Read the model definition and answer for the solid it produces. Units are mm, in the model's axes. Face numbers are marked on the shaded views. A direction names the side the tool comes from. Give positions to 0.01 mm unless a question says otherwise; leave off trailing zeros. Order: outer loops, then holes, each group sorted by start corner. A loop starts at its lowest first (then second) coordinate and runs counter-clockwise, first axis right, second up.
```python
from build123d import *

# Parameters (mm, degrees)
F0_R     = 2.25
F0_R_2   = 33.35
F1_DEPTH = 20
F2_R     = 33.35
F3_DEPTH = 25
F5_DEPTH = 5
F6_R     = 1.49999
F7_SIZE  = 5
F8_R     = 1.99999


# Not quite as in the source:
# - a fillet or chamfer is up to 0.001 mm smaller than in the source, because OpenCascade refuses the exact size


with BuildPart() as f1:
    # F0 (on Top) → F1 (new body)
    with BuildSketch(Plane.XY):
        with BuildLine():
            ThreePointArc((-35.3461431703, -28.7786841774), (-30.3488782685, -27.4389385893), (-25.3508812473, -28.775950375))
            ThreePointArc((-25.3508812473, -28.775950375), (0, -38.35), (25.3508812473, -28.775950375))
            ThreePointArc((25.3508812473, -28.775950375), (30.3488782685, -27.4389385893), (35.3461431703, -28.7786841774))
            ThreePointArc((35.3461431703, -28.7786841774), (45.2498273477, -26.125), (42.5961431703, -16.2213158226))
            ThreePointArc((42.5961431703, -16.2213158226), (38.9372570055, -12.5634302623), (37.5961446665, -7.566531981))
            ThreePointArc((37.5961446665, -7.566531981), (33.2120742351, 19.175), (12.2452634191, 36.342482356))
            ThreePointArc((12.2452634191, 36.342482356), (8.588378737, 40.0023688516), (7.25, 45))
            ThreePointArc((7.25, 45), (5.790617411, 49.3624820917), (2, 51.9686799324))
            Line((2, 51.9686799324), (2, 54.1277186767))
            Line((2, 54.1277186767), (2, 57))
            Line((2, 57), (0, 57))
            Line((0, 57), (-2, 57))
            Line((-2, 57), (-2, 54.1277186767))
            Line((-2, 54.1277186767), (-2, 51.9686799324))
            ThreePointArc((-2, 51.9686799324), (-5.790617411, 49.3624820917), (-7.25, 45))
            ThreePointArc((-7.25, 45), (-8.588378737, 40.0023688516), (-12.2452634191, 36.342482356))
            ThreePointArc((-12.2452634191, 36.342482356), (-33.2120742351, 19.175), (-37.5961446665, -7.566531981))
            ThreePointArc((-37.5961446665, -7.566531981), (-38.9372570055, -12.5634302623), (-42.5961431703, -16.2213158226))
            ThreePointArc((-42.5961431703, -16.2213158226), (-45.2498273477, -26.125), (-35.3461431703, -28.7786841774))
        make_face()
        with Locations((-38.9711431703, -22.5)):
            Circle(F0_R, mode=Mode.SUBTRACT)
        with Locations((38.9711431703, -22.5)):
            Circle(F0_R, mode=Mode.SUBTRACT)
        Circle(F0_R_2, mode=Mode.SUBTRACT)
        with Locations((0, 45)):
            Circle(F0_R, mode=Mode.SUBTRACT)
    extrude(amount=F1_DEPTH)

    # F2 (on Top) → F3 (join)
    with BuildSketch(Plane.XY):
        Polygon((37.0225860118, -21.375), (37.0225860118, 21.375), (0, 42.75), (-37.0225860118, 21.375), (-37.0225860118, -21.375), (0, -42.75), align=None)
        Circle(F2_R, mode=Mode.SUBTRACT)
    extrude(amount=F3_DEPTH)

    # F4 (on face) → F5 (cut)
    with BuildSketch(Plane.XY.offset(25)):
        Polygon((37.0225860118, -21.375), (37.0225860118, 21.375), (0, 42.75), (-37.0225860118, 21.375), (-37.0225860118, -21.375), (0, -42.75), align=None)
        with BuildLine():
            ThreePointArc((-31.7698222916, -16.6102646446), (-31.0470107257, 17.925), (-1.5, 35.8186055005))
            Line((-1.5, 35.8186055005), (-1.5, 38.8186055005))
            Line((-1.5, 38.8186055005), (0, 38.8186055005))
            Line((0, 38.8186055005), (1.5, 38.8186055005))
            Line((1.5, 38.8186055005), (1.5, 35.8186055005))
            ThreePointArc((1.5, 35.8186055005), (31.0470107257, 17.925), (31.7698222916, -16.6102646446))
            Line((31.7698222916, -16.6102646446), (34.3678985029, -18.1102646446))
            Line((34.3678985029, -18.1102646446), (33.6178985029, -19.4093027502))
            Line((33.6178985029, -19.4093027502), (32.8678985029, -20.7083408559))
            Line((32.8678985029, -20.7083408559), (30.2698222916, -19.2083408559))
            ThreePointArc((30.2698222916, -19.2083408559), (0, -35.85), (-30.2698222916, -19.2083408559))
            Line((-30.2698222916, -19.2083408559), (-32.8678985029, -20.7083408559))
            Line((-32.8678985029, -20.7083408559), (-33.6178985029, -19.4093027502))
            Line((-33.6178985029, -19.4093027502), (-34.3678985029, -18.1102646446))
            Line((-34.3678985029, -18.1102646446), (-31.7698222916, -16.6102646446))
        make_face(mode=Mode.SUBTRACT)
    extrude(amount=-F5_DEPTH, mode=Mode.SUBTRACT)

    # F6 (radius 1.5 in the source; OpenCascade refuses exactly that, so slightly less here)
    f6_edges = [f1.edges().sort_by_distance(p)[0] for p in [
        (-32.867899, -20.708341, 22.5),
        (-34.367899, -18.110265, 22.5),
        (32.867899, -20.708341, 22.5),
        (34.367899, -18.110265, 22.5),
        (1.5, 38.818606, 22.5),
        (-1.5, 38.818606, 22.5),
    ]]
    fillet(f6_edges, radius=F6_R)

    # F7
    f7_edges = [f1.edges().sort_by_distance(p)[0] for p in [
        (0, -42.75, 10),
        (37.022586, 21.375, 10),
        (-37.022586, 21.375, 10),
    ]]
    chamfer(f7_edges, length=F7_SIZE)

    # F8 (radius 2 in the source; OpenCascade refuses exactly that, so slightly less here)
    f8_edges = [f1.edges().sort_by_distance(p)[0] for p in [
        (-2, 57, 10),
        (2, 57, 10),
        (-2, 51.96868, 10),
        (2, 51.96868, 10),
    ]]
    fillet(f8_edges, radius=F8_R)


solid = f1.part
```
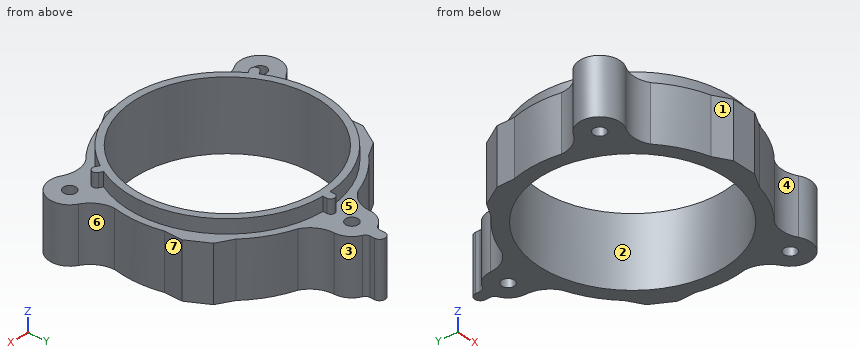
1) Given pin 1 (0.5 mm diameter, centred on y = 36.5, z = 23, fed in from -X); pin 2 (1 mm diameter, centred on y = 12.5, z = 21, fed in from +X); pin 3 (3 mm diameter, centred on y = 13.5, z = 13, fed in from +X); pin 4 (3.5 mm diameter, centred on x = 0, y = 45, fed in from -Z), each flat-ended and moving along its own axis, determine where each tip first touches the part or whether it passes through.
Final values:
pin 1: stops at x = -1.5
pin 2: stops at x = 33.78
pin 3: stops at x = 37.02
pin 4: passes through
2) For a pull along X with two mould halves and no side action, classify the marked faces 1, 2, 3 and 4 as released by +X, released by -X, zero draft, split by the parting line, or undercut.
Final values:
face 1: released by -X
face 2: undercut
face 3: released by +X
face 4: undercut
3) The part is cut by section D-D on y = 32. Determine the outline of the cut face in (x, z).
Final values:
outline: (-21.14, 0) - (-9.39, 0) - (-9.39, 25) - (-16.16, 25) - (-16.16, 20) - (-21.14, 20) - close; (9.39, 0) - (21.14, 0) - (21.14, 20) - (16.16, 20) - (16.16, 25) - (9.39, 25) - close
4) A tool of negligible diameter and unlimited length cuts with its end or side. For the marked faces 5, 6 and 7, from which of +Z, -Z, +X, -X, +Y, -Y can it reach the whole face along a straight path? Write none if from no direction.
Final values:
face 5: +Z
face 6: +Z, -Z, +X
face 7: +Z, -Z, +X, +Y
5) The part is cut by section C-C on z = 6.25. Count the separate pieces of the cut face and the enclosed holes in it, and give its area (3 significant figures).
Final values:
separate pieces: 1
enclosed holes: 4
area: 1,780 mm2
6) The part is cut by section A-A on y = 0. Determine the outline of the cut face in (x, z), and give its area (3 significant figures).
Final values:
outline: (-38.35, 0) - (-33.35, 0) - (-33.35, 25) - (-35.85, 25) - (-35.85, 20) - (-38.35, 20) - close; (33.35, 0) - (38.35, 0) - (38.35, 20) - (35.85, 20) - (35.85, 25) - (33.35, 25) - close
area: 225 mm2
7) The part is cut by section B-B on y = -22.5. Determine the outline of the cut face in (x, z), and give its area (3 significant figures).
Final values:
outline: (-46.22, 0) - (-41.22, 0) - (-41.22, 20) - (-46.22, 20) - close; (-36.72, 0) - (-24.62, 0) - (-24.62, 25) - (-27.91, 25) - (-27.91, 20) - (-36.72, 20) - close; (24.62, 0) - (36.72, 0) - (36.72, 20) - (27.91, 20) - (27.91, 25) - (24.62, 25) - close; (41.22, 0) - (46.22, 0) - (46.22, 20) - (41.22, 20) - close
area: 717 mm2
8) Consider L1, parallel to X at y = -1, z = 5.5 (3 decimals); L2, parallel to Y at x = 0, z = 12.75; L3, parallel to Y at x = -0.5, z = 5. Determine where each line is inside the solid, lowest interval first.
Final values:
L1: x = -38.337 to -33.335, 33.335 to 38.337
L2: y = -40.25 to -33.35, 33.35 to 42.75, 47.25 to 57
L3: y = -40.25 to -33.35, 33.35 to 42.81, 47.19 to 56.94
